CAD build for the part. Positions are in the model's coordinates, mm. A direction names the side the tool comes from. Round coordinates to 2 decimals unless told otherwise and drop trailing zeros. Order: outer loops, then holes, each group sorted by start corner. A loop starts at its lowest first (then second) coordinate and runs counter-clockwise, first axis right, second up. Notation, with made-up numbers: M 79,39.5 L 103,39.5 A9 ccw 103,55.5 Z; hole C 78,75.5 d6. An arc over 180 degrees is marked long. Put each result on its own line as item: value.
```python
from build123d import *

# Parameters (mm, degrees)
SKETCH_1_R      = 1.75
SKETCH_1_W      = 14.344262296
SKETCH_1_H      = 5.737704918
SKETCH_1_W_2    = 14.344262295
SKETCH_1_W_3    = 47.62295082
SKETCH_1_H_2    = 24.672131148
EXTRUDE_1_DEPTH = 3


with BuildPart() as part:
    # 草图1 → 凸台-拉伸1 (new body)
    with BuildSketch(Plane.XZ):
        with BuildLine():
            Line((-27.944138099, -25.958892198), (-33.179876582, -31.19463068))
            ThreePointArc((-33.179876582, -31.19463068), (-33.926143431, -32.311497947), (-34.188197499, -33.628932714))
            Line((-34.188197499, -33.628932714), (-34.188197499, -40.293115532))
            ThreePointArc((-34.188197499, -40.293115532), (-33.179876582, -42.727417565), (-30.745574548, -43.735738483))
            Line((-30.745574548, -43.735738483), (-24.08139173, -43.735738483))
            ThreePointArc((-24.08139173, -43.735738483), (-22.763956963, -43.473684414), (-21.647089697, -42.727417565))
            Line((-21.647089697, -42.727417565), (-10.969266445, -32.049594314))
            ThreePointArc((-10.969266445, -32.049594314), (-7.246375557, -29.562038152), (-2.854926333, -28.68852459))
            Line((-2.854926333, -28.68852459), (23.097549284, -28.68852459))
            ThreePointArc((23.097549284, -28.68852459), (27.488998508, -29.562038152), (31.211889396, -32.049594314))
            Line((31.211889396, -32.049594314), (41.889712647, -42.727417565))
            ThreePointArc((41.889712647, -42.727417565), (43.006579914, -43.473684414), (44.324014681, -43.735738483))
            Line((44.324014681, -43.735738483), (50.988197499, -43.735738483))
            ThreePointArc((50.988197499, -43.735738483), (53.422499533, -42.727417565), (54.43082045, -40.293115532))
            Line((54.43082045, -40.293115532), (54.43082045, -33.628932714))
            ThreePointArc((54.43082045, -33.628932714), (54.168766382, -32.311497947), (53.422499533, -31.19463068))
            Line((53.422499533, -31.19463068), (42.802053331, -20.574184478))
            ThreePointArc((42.802053331, -20.574184478), (40.314497168, -16.85129359), (39.440983607, -12.459844366))
            Line((39.440983607, -12.459844366), (39.440983607, 12.459844366))
            ThreePointArc((39.440983607, 12.459844366), (40.314497168, 16.85129359), (42.802053331, 20.574184478))
            Line((42.802053331, 20.574184478), (53.422499533, 31.19463068))
            ThreePointArc((53.422499533, 31.19463068), (54.168766382, 32.311497947), (54.43082045, 33.628932714))
            Line((54.43082045, 33.628932714), (54.43082045, 40.293115532))
            ThreePointArc((54.43082045, 40.293115532), (53.422499533, 42.727417565), (50.988197499, 43.735738483))
            Line((50.988197499, 43.735738483), (44.324014681, 43.735738483))
            ThreePointArc((44.324014681, 43.735738483), (43.006579914, 43.473684414), (41.889712647, 42.727417565))
            Line((41.889712647, 42.727417565), (31.211889396, 32.049594314))
            ThreePointArc((31.211889396, 32.049594314), (27.488998508, 29.562038152), (23.097549284, 28.68852459))
            Line((23.097549284, 28.68852459), (-2.854926333, 28.68852459))
            ThreePointArc((-2.854926333, 28.68852459), (-7.246375557, 29.562038152), (-10.969266445, 32.049594314))
            Line((-10.969266445, 32.049594314), (-21.647089697, 42.727417565))
            ThreePointArc((-21.647089697, 42.727417565), (-22.763956963, 43.473684414), (-24.08139173, 43.735738483))
            Line((-24.08139173, 43.735738483), (-30.745574548, 43.735738483))
            ThreePointArc((-30.745574548, 43.735738483), (-33.179876582, 42.727417565), (-34.188197499, 40.293115532))
            Line((-34.188197499, 40.293115532), (-34.188197499, 33.628932714))
            ThreePointArc((-34.188197499, 33.628932714), (-33.926143431, 32.311497947), (-33.179876582, 31.19463068))
            Line((-33.179876582, 31.19463068), (-27.944138099, 25.958892198))
            ThreePointArc((-27.944138099, 25.958892198), (-27.180473754, 22.249967152), (-30.286027184, 20.083207792))
            ThreePointArc((-30.286027184, 20.083207792), (-32.264648538, 19.216561535), (-33.077868852, 17.215389149))
            Line((-33.077868852, 17.215389149), (-33.077868852, -17.215389149))
            ThreePointArc((-33.077868852, -17.215389149), (-32.264648538, -19.216561535), (-30.286027184, -20.083207792))
            ThreePointArc((-30.286027184, -20.083207792), (-27.180473754, -22.249967152), (-27.944138099, -25.958892198))
        make_face()
        with Locations(Location((48.664427007, 38.543115532, 0), (0, 0, 90))):
            Circle(SKETCH_1_R, mode=Mode.SUBTRACT)
        with Locations(Location((-28.421804056, -38.543115532, 0), (0, 0, 90))):
            Circle(SKETCH_1_R, mode=Mode.SUBTRACT)
        with Locations(Location((27.885245902, 5.594262295, 0), (0, 0, 90))):
            Circle(SKETCH_1_R, mode=Mode.SUBTRACT)
        with Locations(Location((-27.885245902, 5.594262295, 0), (0, 0, 90))):
            Circle(SKETCH_1_R, mode=Mode.SUBTRACT)
        with Locations(Location((-27.885245902, -5.594262295, 0), (0, 0, 90))):
            Circle(SKETCH_1_R, mode=Mode.SUBTRACT)
        with Locations(Location((27.885245902, -5.594262295, 0), (0, 0, 90))):
            Circle(SKETCH_1_R, mode=Mode.SUBTRACT)
        with Locations(Location((48.664427007, -38.543115532, 0), (0, 0, 90))):
            Circle(SKETCH_1_R, mode=Mode.SUBTRACT)
        with Locations(Location((-28.421804056, 38.543115532, 0), (0, 0, 90))):
            Circle(SKETCH_1_R, mode=Mode.SUBTRACT)
        with Locations((25.9, -20.368852459)):
            Rectangle(SKETCH_1_W, SKETCH_1_H, mode=Mode.SUBTRACT)
        with Locations((-5.65737705, 20.368852459)):
            Rectangle(SKETCH_1_W_2, SKETCH_1_H, mode=Mode.SUBTRACT)
        Rectangle(SKETCH_1_W_3, SKETCH_1_H_2, mode=Mode.SUBTRACT)
        with Locations((25.9, 20.368852459)):
            Rectangle(SKETCH_1_W, SKETCH_1_H, mode=Mode.SUBTRACT)
        with Locations((-5.65737705, -20.368852459)):
            Rectangle(SKETCH_1_W_2, SKETCH_1_H, mode=Mode.SUBTRACT)
    extrude(amount=-EXTRUDE_1_DEPTH)


solid = part.part
```
Item 1: Band-saw the part on A-A on z = 30. Give the cut face in (x, y), and give its area (3 significant figures).
Answers below:
outline: M -31.99,0 L -8.18,0 L -8.18,3 L -31.99,3 Z; M 28.42,0 L 52.23,0 L 52.23,3 L 28.42,3 Z
area: 143 mm²
Item 2: Tool access for faces 1 (the cylindrical face through (43.02, 1.48, 43.48)), 2 (the flat face through (26, 1, 23.238)), 3 (the flat face through (10, 1, -28.689)), 4 (the flat face through (48.19, 1.48, -25.96)), 5 (the cylindrical face through (-33.919, 1.479, -32.294)): list every direction of +Z, -Z, +X, -X, +Y, -Y with a clear straight run to the whole face (end or side of a thin tool).
Answers below:
face 1: +Z, +Y, -Y
face 2: +Y, -Y
face 3: -Z, +Y, -Y
face 4: +X, +Y, -Y
face 5: -X, +Y, -Y
Item 3: Mould opens along Z. For faces 6 (the cylindrical face through (42.989, 1.479, -43.466)), 7 (the cylindrical face through (-33.153, 1.479, 42.754)), 8 (the cylindrical face through (28.56, 1.48, -3.98)) say: pulls with the +Z half, pulls with the -Z half, needs draft (parallel to the pull), parting line crosses it, or undercut.
Answers below:
face 6: pulls with the -Z half
face 7: pulls with the +Z half
face 8: undercut
Item 4: Pin check, flat tips, straight feed: P1, Ø0.9, axis at x = 29, y = 2, coming from the +Z side; P2, Ø0.9, axis at y = 2, z = -3.5, coming from the -X side; P3, Ø6, axis at x = 20, z = -7, coming from the -Y side; P4, Ø1.5, axis at x = -8.5, y = 2, coming from the -Z side. Stop position of each tip, or through.
Answers below:
P1: z = 30.61
P2: x = -33.08
P3: through
P4: z = -30.64
Item 5: Band-saw the part on C-C on z = -15.5. Give the cut face in (x, y).
Answers below:
outline: M -33.08,0 L 39.85,0 L 39.85,3 L -33.08,3 Z
Item 6: Probe line 1 along X through (y, z) = (2.1, -5.5); line 2 along Z through (x, y) = (23.5, 2.65); line 3 along Z through (x, y) = (24.5, 2.5). List the from-to ranges inside material, lowest first. Write a range as [from, to].
Answers below:
line 1: [-33.08, -29.63], [-26.14, -23.81], [23.81, 26.14], [29.63, 39.44]
line 2: [-28.7, -23.24], [-17.5, -12.34], [12.34, 17.5], [23.24, 28.7]
line 3: [-28.77, -23.24], [-17.5, 17.5], [23.24, 28.77]
Item 7: Band-saw the part on B-B on y = 0.5. State how many separate pieces and enclosed holes the cut face has, and give its area (3 significant figures).
Answers below:
separate pieces: 1
enclosed holes: 13
area: 3,750 mm²
